Answer from the drawing. Dimensions are ordinates in mm from the lowest x, y and z of the part. A direction names the side the tool comes from. Give positions to 0.01 mm unless a question says otherwise; leave off trailing zeros. Write each loop counter-clockwise with the first axis right and the second up, starting at its lowest first coordinate (ties: lowest second). Pieces come first, ordered by that corner, then holes.
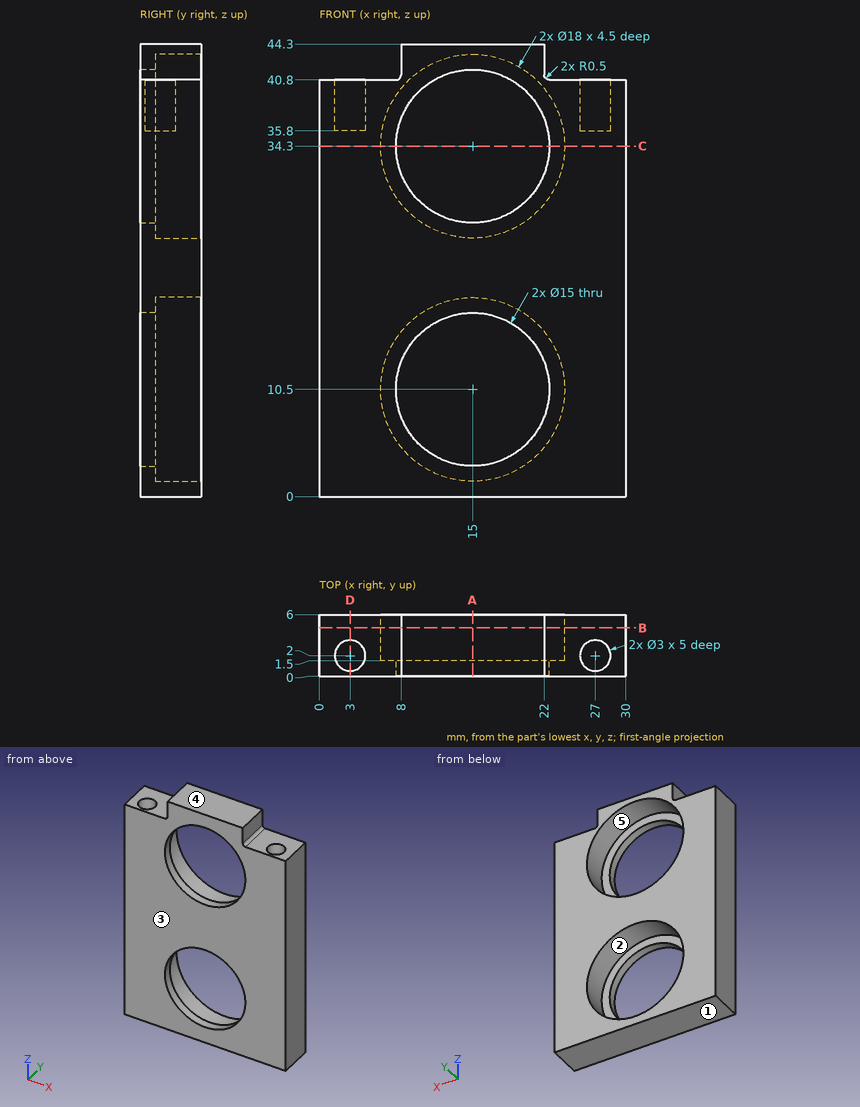
Item 1: Each of these flat-tipped pins is pushed along its axis until it touches: P1, Ø1.5, axis at x = 26, y = 5, coming from the +Z side; P2, Ø2.5, axis at x = 27, y = 2, coming from the -Z side; P3, Ø2.5, axis at x = 3, y = 2, coming from the +Z side; P4, Ø2.5, axis at y = 4.5, z = 43, coming from the -X side. Where does it stop, or does it pass through?
Conclusion:
P1: stops at z = 40.8
P2: stops at z = 0
P3: stops at z = 35.8
P4: stops at x = 8
Item 2: Which of the six approach directions +Z, -Z, +X, -X, +Y, -Y give full straight-line access (tool end or side, diameter ignored) to the marked faces 1 and 2?
Conclusion:
face 1: -Z, +X, -X, +Y, -Y
face 2: +Y
Item 3: A cutting plane is placed at C-C, the plane z = 34.3. Give the vertices of the cut face in (x, y), plus the area to 3 significant figures.
Conclusion:
outline: (0, 0) - (7.5, 0) - (7.5, 1.5) - (6, 1.5) - (6, 6) - (0, 6) - close; (22.5, 0) - (30, 0) - (30, 6) - (24, 6) - (24, 1.5) - (22.5, 1.5) - close
area: 76.5 mm2
Item 4: A cutting plane is placed at A-A, the plane x = 15. Give the vertices of the cut face in (y, z), plus the area to 3 significant figures.
Conclusion:
outline: (0, 0) - (6, 0) - (6, 1.5) - (1.5, 1.5) - (1.5, 3) - (0, 3) - close; (0, 18) - (1.5, 18) - (1.5, 19.5) - (6, 19.5) - (6, 25.3) - (1.5, 25.3) - (1.5, 26.8) - (0, 26.8) - close; (0, 41.8) - (1.5, 41.8) - (1.5, 43.3) - (6, 43.3) - (6, 44.3) - (0, 44.3) - close
area: 58.8 mm2
Item 5: A cutting plane is placed at D-D, the plane x = 3. Give the vertices of the cut face in (y, z), plus the area to 3 significant figures.
Conclusion:
outline: (0, 0) - (6, 0) - (6, 40.8) - (3.5, 40.8) - (3.5, 35.8) - (0.5, 35.8) - (0.5, 40.8) - (0, 40.8) - close
area: 230 mm2
Item 6: A cutting plane is placed at B-B, the plane y = 4.7. Give the vertices of the cut face in (x, z), plus the area to 3 significant figures.
Conclusion:
outline: (0, 0) - (30, 0) - (30, 40.8) - (22.5, 40.8) arc R0.5 cw to (22, 41.3) - (22, 44.3) - (8, 44.3) - (8, 41.3) arc R0.5 cw to (7.5, 40.8) - (0, 40.8) - close; hole circle Ø18 at (15, 10.5); hole circle Ø18 at (15, 34.3)
area: 764 mm2
Item 7: Determine the mould class of the marked faces 3, 4 and 5 for opening direction Z: pulls with the +Z half, pulls with the -Z half, needs draft (parallel to the pull), parting line crosses it, or undercut.
Conclusion:
face 3: needs draft
face 4: pulls with the +Z half
face 5: undercut
Item 8: Consider probe 1 along X at (y, z) = (1.2, 10.5); probe 2 along Z at (x, y) = (11.75, 3.75); probe 3 along X at (y, z) = (2.2, 34) (3 decimals). Determine where each line is inside the solid, lowest interval first.
Conclusion:
probe 1: x = 0 to 7.5, 22.5 to 30
probe 2: z = 0 to 2.11, 18.89 to 25.91, 42.69 to 44.3
probe 3: x = 0 to 6.005, 23.995 to 30
